```python
from build123d import *

# Parameters (mm, degrees)
F0_R     = 1.5
F1_DEPTH = 3.175
F0_W     = 3.175
F0_H     = 3.175
F2_DEPTH = 12.7


with BuildPart() as f1:
    # F0 (on Front) → F1 (new body)
    with BuildSketch(Plane.XZ):
        with BuildLine():
            Line((-91.283362, -36.782738), (-91.283362, 26.717262))
            ThreePointArc((-91.283362, 26.717262), (-96.839612, 43.97878), (-102.395862, 26.717262))
            Line((-102.395862, 26.717262), (-102.395862, -36.782738))
            Line((-102.395862, -36.782738), (-99.220862, -36.782738))
            Line((-99.220862, -36.782738), (-94.458362, -36.782738))
            Line((-94.458362, -36.782738), (-91.283362, -36.782738))
        make_face()
        with Locations((-96.839612, 34.45378)):
            Circle(F0_R, mode=Mode.SUBTRACT)
    extrude(amount=F1_DEPTH)

    # F0 (on Front) → F2 (join)
    with BuildSketch(Plane.XZ):
        with Locations((-100.808362, -38.370238)):
            Rectangle(F0_W, F0_H)
        with Locations((-92.870862, -38.370238)):
            Rectangle(F0_W, F0_H)
    extrude(amount=F2_DEPTH)


solid = f1.part
```
Design review of the part built by this model. Coordinates are the model's own, in mm. A direction names the side the tool comes from. Round coordinates to 2 decimals unless told otherwise and drop trailing zeros. Write each loop counter-clockwise with the first axis right and the second up, starting at its lowest first coordinate (ties: lowest second). Pieces come first, ordered by that corner, then holes. Notation, with made-up numbers: (-23.5, 38.5) -> (-12.5, 38.5) arc R33 ccw to (-12.5, 70.5) -> close; hole circle Ø1 at (44, 59). An arc over 180 degrees is marked (long way). Answer in a Markdown table with one row per item.
Q1. To check wall thickness, follow L1, parallel to Y at x = -92, z = -3 (3 decimals); L2, parallel to Z at x = -100.75, y = -11.5; L3, parallel to X at y = -0.75, z = 21. State the ranges of each line that lie inside material, in increasing order. Write a range as [from, to].
The answers:
| item | result |
|---|---|
| L1 | [-3.175, 0] |
| L2 | [-39.96, -36.78] |
| L3 | [-102.4, -91.28] |
Q2. Clearance check with flat-ended pins moving along their axes: pin 1 Ø1 at (x, z) = (-97.5, 33) entering from -Y (3 decimals); pin 2 Ø1 at (y, z) = (-4, -38.5) entering from -X; pin 3 Ø1.6 at (x, y) = (-92.5, -9) entering from +Z. State where each tip first meets the part, or that it passes through.
The answers:
| item | result |
|---|---|
| pin 1 | y = -3.175 |
| pin 2 | x = -102.4 |
| pin 3 | z = -36.78 |
Q3. Draft analysis for pull direction Z (two halves, no side actions). For faces 6 (the face through (-95.454, -1.565, 33.879)), 7 (the face through (-93, -12.7, -38)), 8 (the face through (-93, -6, -39.958)), 9 (the face through (-93, -8, -36.783)), state which applies: +Z half, -Z half, draft (parallel to the pull), parting line (faces both ways), or undercut.
The answers:
| item | result |
|---|---|
| face 6 | undercut |
| face 7 | draft |
| face 8 | -Z half |
| face 9 | +Z half |
Q4. Take a section at C-C, the plane y = -1.5. State the section outline as (x, z) points (3 decimals), then the cut area to 3 significant figures.
The answers:
| item | result |
|---|---|
| outline | (-102.396, -39.958) -> (-99.221, -39.958) -> (-99.221, -36.783) -> (-94.458, -36.783) -> (-94.458, -39.958) -> (-91.283, -39.958) -> (-91.283, 26.717) arc R9.525 ccw (long way) to (-102.396, 26.717) -> close; hole circle Ø3 at (-96.84, 34.454) |
| area | 990 mm² |
Q5. Take a section at D-D, the plane x = -93.5. State the section outline as (y, z) points (3 decimals), then the cut area to 3 significant figures.
The answers:
| item | result |
|---|---|
| outline | (-12.7, -39.958) -> (0, -39.958) -> (0, 43.374) -> (-3.175, 43.374) -> (-3.175, -36.783) -> (-12.7, -36.783) -> close |
| area | 295 mm² |
Q6. For faces 1 (the face through (-101, -8, -36.783)), 2 (the face through (-91.283, -3, -9)), 3 (the face through (-102.396, -3, -9)), 4 (the face through (-99.221, -6, -38)), 5 (the face through (-101, -6, -39.958)), list the 3-axis set-ups (+Z, -Z, +X, -X, +Y, -Y) from which the entire face can be reached by the end or side of a thin tool; tool diameter is ignored.
The answers:
| item | result |
|---|---|
| face 1 | +Z, +X, -X, -Y |
| face 2 | -Z, +X, +Y, -Y |
| face 3 | -Z, -X, +Y, -Y |
| face 4 | -Z, +Y, -Y |
| face 5 | -Z, +X, -X, +Y, -Y |
Q7. Take a section at B-B, the plane x = -97.25. State the section outline as (y, z) points (3 decimals).
The answers:
| item | result |
|---|---|
| outline | (-3.175, -36.783) -> (0, -36.783) -> (0, 33.011) -> (-3.175, 33.011) -> close; (-3.175, 35.897) -> (0, 35.897) -> (0, 43.97) -> (-3.175, 43.97) -> close |
Q8. Take a section at A-A, the plane y = -9.75. State the section outline as (x, z) points, then the cut area to 3 significant figures.
The answers:
| item | result |
|---|---|
| outline | (-102.4, -39.96) -> (-99.22, -39.96) -> (-99.22, -36.78) -> (-102.4, -36.78) -> close; (-94.46, -39.96) -> (-91.28, -39.96) -> (-91.28, -36.78) -> (-94.46, -36.78) -> close |
| area | 20.2 mm² |
